Here's the drawing with two shaded views (mm, measured from the low corner). I have some questions. A direction names the side the tool comes from. Give positions to 0.01 mm unless a question says otherwise; leave off trailing zeros. Write each loop counter-clockwise with the first axis right and the second up, starting at its lowest first coordinate (ties: lowest second). Pieces come first, ordered by that corner, then holes. Notation, with made-up numbers: (64.5, 16.25) - (111.5, 16.25) arc R8 cw to (111.5, 24.25) - close; hole circle Ø10 at (85, 8). An arc over 180 degrees is marked (long way). Answer as a JSON object with one key per item and string values. Group by question number.
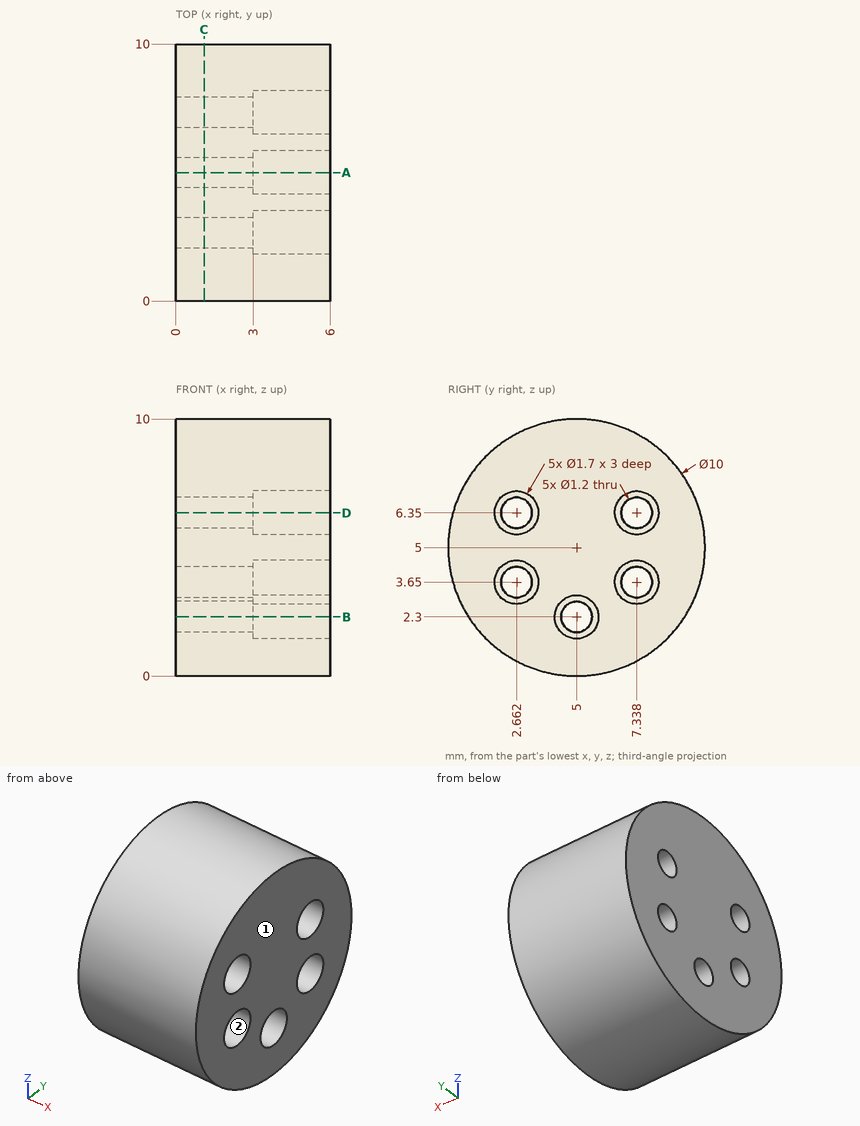
(1) I want a section at B-B, the plane z = 2.3. Please give me the cut outline in (x, y), and give its area (3 significant figures).
(2) Will these pins go through, and if not, where does the flat tip stop? P1, Ø0.8, axis at y = 2.5, z = 6, coming from the +X side; P2, Ø1.5, axis at x = 5, z = 1.5, coming from the +Y side (1 decimal).
(3) I want a section at A-A, the plane y = 5. Please give me the cut outline in (x, z).
(4) I want a section at D-D, the plane z = 6.35. Please give me the cut outline in (x, y).
(5) For the marked faces 1 and 2, which set-ups out of +Z, -Z, +X, -X, +Y, -Y let a thin tool reach every point of the face, with its end or its side?
(6) I need wall thicknesses on L1, parallel to Z at x = 0.55, y = 7.75 (1 decimal); L2, parallel to Y at x = 4, z = 6.35 (1 decimal); L3, parallel to Z at x = 4.65, y = 5. Which ranges of each line are inside material? Lowest first, please.
(7) I want a section at C-C, the plane x = 1.1. Please give me the cut outline in (y, z).
Entries:
{
 "1": {"outline": "(0, 0.79) - (6, 0.79) - (6, 4.15) - (3, 4.15) - (3, 4.4) - (0, 4.4) - close; (0, 5.6) - (3, 5.6) - (3, 5.85) - (6, 5.85) - (6, 9.21) - (0, 9.21) - close", "area": "41.8 mm^2"},
 "2": {"P1": "x = 3", "P2": "y = 9.2"},
 "3": {"outline": "(0, 0) - (6, 0) - (6, 1.45) - (3, 1.45) - (3, 1.7) - (0, 1.7) - close; (0, 2.9) - (3, 2.9) - (3, 3.15) - (6, 3.15) - (6, 10) - (0, 10) - close"},
 "4": {"outline": "(0, 0.19) - (6, 0.19) - (6, 1.81) - (3, 1.81) - (3, 2.06) - (0, 2.06) - close; (0, 3.26) - (3, 3.26) - (3, 3.51) - (6, 3.51) - (6, 6.49) - (3, 6.49) - (3, 6.74) - (0, 6.74) - close; (0, 7.94) - (3, 7.94) - (3, 8.19) - (6, 8.19) - (6, 9.81) - (0, 9.81) - close"},
 "5": {"face 1": "+Z, -Z, +X, +Y, -Y", "face 2": "+X"},
 "6": {"L1": "0.8 to 3.2, 4.1 to 5.9, 6.8 to 9.2", "L2": "0.2 to 1.8, 3.5 to 6.5, 8.2 to 9.8", "L3": "0 to 1.45, 3.15 to 10"},
 "7": {"outline": "circle Ø10 at (5, 5); hole circle Ø1.2 at (2.66, 3.65); hole circle Ø1.2 at (2.66, 6.35); hole circle Ø1.2 at (5, 2.3); hole circle Ø1.2 at (7.34, 3.65); hole circle Ø1.2 at (7.34, 6.35)"}
}
